```python
from build123d import *

# Parameters (mm, degrees)
SKETCH1_W           = 19.05
SKETCH1_H           = 9.525
BOSS_EXTRUDE1_DEPTH = 6.35
BOSS_EXTRUDE2_START = 1.5875
BOSS_EXTRUDE2_DEPTH = 3.175
SKETCH3_R           = 1.27
CUT_EXTRUDE1_DEPTH  = 59.227939899


with BuildPart() as part:
    # Sketch1 → Boss-Extrude1 (new body)
    with BuildSketch(Plane.XY):
        with Locations((9.525, 4.7625)):
            Rectangle(SKETCH1_W, SKETCH1_H)
    extrude(amount=BOSS_EXTRUDE1_DEPTH)

    # Sketch2 → Boss-Extrude2 (add)
    with BuildSketch(Plane.XY.offset(BOSS_EXTRUDE2_START)):
        Polygon((0.875640633, 9.525), (53.247352459, 22.582734315), (53.29343858, 22.397892979), (1.66308486, 9.525), align=None)
    extrude(amount=BOSS_EXTRUDE2_DEPTH)

    # Sketch3 → Cut-Extrude1 (cut, through all)
    with BuildSketch(Plane.XY.offset(6.35)):
        with Locations((4.445, 2.06375)):
            Circle(SKETCH3_R)
        with Locations(Location((14.605, 2.06375, 0), (0, 0, 180))):
            Circle(SKETCH3_R)
    extrude(amount=-CUT_EXTRUDE1_DEPTH, mode=Mode.SUBTRACT)


solid = part.part
```
Check sheet for the modelled part. Datum: model origin and axes. Units: mm. Round coordinates to 2 decimals unless told otherwise and drop trailing zeros. Loops run counter-clockwise (first coordinate to the right, second up) from the corner with the lowest first, then second, coordinate; pieces in that order, holes last. Notation, with made-up numbers: (34, 49.25) -> (85, 49.25) arc R8 ccw to (85, 57.25) -> close; hole circle Ø10 at (36, 7). An arc over 180 degrees is marked (long way). Answer in a Markdown table with one row per item.
Q1. Thickness scan on L1, parallel to X at y = 9, z = 4.75; L2, parallel to X at y = 1, z = 0.75; L3, parallel to Y at x = 7.5, z = 2.5 (3 decimals). Record the ranges inside material, lowest first.
Data:
| item | result |
|---|---|
| L1 | x = 0 to 19.05 |
| L2 | x = 0 to 3.75, 5.14 to 13.91, 15.3 to 19.05 |
| L3 | y = 0 to 9.525, 10.98 to 11.177 |
Q2. Sectioned sample at B-B on x = 4.5. Give the number of separate pieces and of enclosed holes in the cut face, then the cut area to 3 significant figures.
Data:
| item | result |
|---|---|
| separate pieces | 3 |
| enclosed holes | 0 |
| area | 45.0 mm^2 |
Q3. Sectioned sample at D-D on y = 8. Enter the section's corners in (x, z).
Data:
| item | result |
|---|---|
| outline | (0, 0) -> (19.05, 0) -> (19.05, 6.35) -> (0, 6.35) -> close |
Q4. Sectioned sample at C-C on z = 2.5. Enter the section's corners in (x, y) (3 decimals), then the cut area to 3 significant figures.
Data:
| item | result |
|---|---|
| outline | (0, 0) -> (19.05, 0) -> (19.05, 9.525) -> (1.663, 9.525) -> (53.293, 22.398) -> (53.247, 22.583) -> (0.876, 9.525) -> (0, 9.525) -> close; hole circle Ø2.54 at (4.445, 2.064); hole circle Ø2.54 at (14.605, 2.064) |
| area | 182 mm^2 |
Q5. Release check for a two-part mould opening along Y. For faces 1 (the face through (19.05, 5, 3)), 2 (the face through (13.43, 2.55, 3.22)), 3 (the face through (27.84, 16.05, 3.15)), 4 (the face through (9, 0, 3)) record: released by +Y, released by -Y, zero draft, split by the parting line, or undercut.
Data:
| item | result |
|---|---|
| face 1 | zero draft |
| face 2 | undercut |
| face 3 | undercut |
| face 4 | released by -Y |
Q6. Go/stop test with flat-tipped pins: P1, Ø3, axis at x = 21, z = 1, coming from the +Y side; P2, Ø10.5, axis at x = 19, y = 14.5, coming from the +Z side; P3, Ø2, axis at x = 22, z = 3, coming from the -Y side; P4, Ø1.9, axis at x = 10.5, z = 3.5, coming from the +Y side. Record where each tip stops, or that it passes through.
Data:
| item | result |
|---|---|
| P1 | stops at y = 14.89 |
| P2 | stops at z = 6.35 |
| P3 | stops at y = 14.35 |
| P4 | stops at y = 12.16 |
